The model under review builds one solid part; all positions refer to its coordinate system, in mm. A direction names the side the tool comes from. Round coordinates to 2 decimals unless told otherwise and drop trailing zeros. Order: outer loops, then holes, each group sorted by start corner. A loop starts at its lowest first (then second) coordinate and runs counter-clockwise, first axis right, second up. Notation, with made-up numbers: M -3,60.25 L 25,60.25 A31 ccw 25,93.25 Z; hole C 8.25,63 d10. An arc over 180 degrees is marked long. Use a Markdown table: item, result. Add a question column.
1. Consider section A-A on z = 5.08. Count the separate pieces of the cut face and the enclosed holes in it, then the cut area to 3 significant figures.
2. Consider section D-D on y = -3.25. State the section outline as (x, z) points, then the cut area to 3 significant figures.
3. For faces 1 (the flat face through (-5.5, 6.1, 0)), 2 (the flat face through (-18, 5.913, 10)), 3 (the flat face through (-18, 5.913, 1)), list the 3-axis set-ups (+Z, -Z, +X, -X, +Y, -Y) from which the entire face can be reached by the end or side of a thin tool; tool diameter is ignored.
4. Insertion check: P1, Ø6, axis at y = -3, z = 7, coming from the -X side; P2, Ø5, axis at x = -12, y = 2, coming from the +Z side; P3, Ø3, axis at y = 4, z = 5, coming from the -X side; P4, Ø1, axis at y = 1, z = 3, coming from the -X side. Each pin has a flat end and moves straight along its axis. Give the tip position at first contact, or say it passes through.
5. To check wall thickness, follow probe 1 along Y at (x, z) = (-2, 8); probe 2 along Y at (x, z) = (4, 1); probe 3 along X at (y, z) = (0, 0.5). State the ranges of each line that lie inside material, in increasing order.
6. Consider section B-B on y = 3. State the section outline as (x, z) points, then the cut area to 3 significant figures.
7. Consider section C-C on x = -1.5. State the section outline as (y, z) points, then the cut area to 3 significant figures.
8. The part is to be moulded in two halves that separate along X. For faces 4 (the cylindrical face through (5.74, 0.44, 5.01)), 5 (the flat face through (-18, -5.298, 1)), 6 (the cylindrical face through (5.38, 0.43, 5.01)), say which applies: +X half, -X half, draft (parallel to the pull), parting line (faces both ways), or undercut.
Autodesk Inventor part; units mm, degrees
ref_plane "YZ Plane" through (0, 0, 0) normal (1, 0, 0) x (0, 1, 0)
ref_plane "XZ Plane" through (0, 0, 0) normal (0, 1, 0) x (-1, 0, 0)
ref_plane "XY Plane" through (0, 0, 0) normal (0, 0, 1) x (1, 0, 0)
sketch "Sketch1" plane through (0, 0, 0) normal (0, 0, 1) x (1, 0, 0)
  arc A0 (0, -5.6567) -> (0, 6.271) centre (-0.2268, 0.3072) ccw
  line L0 (0, 6.271) -> (-18.4804, 6.271)
  line L1 (0, -5.6567) -> (-18.4804, -5.6567)
  line L2 (-18.122, 5.9127) -> (-0.0069, 5.9127)
  arc A1 (-0.0069, -5.2984) -> (-0.0069, 5.9127) centre (-0.2268, 0.3072) ccw
  line L3 (-0.0069, -5.2984) -> (-18.122, -5.2984)
  line L4 (-18.122, 5.9127) -> (-18.4804, 5.9127)
  line L5 (-18.4804, 6.271) -> (-18.4804, 5.9127)
  line L6 (-18.122, -5.2984) -> (-18.4804, -5.2984)
  line L7 (-18.4804, -5.6567) -> (-18.4804, -5.2984)
  point P0 (0, 0)
extrude "Extrusion1" add sketch "Sketch1" along normal blind 10.16
sketch "Sketch2" plane through (-18.4804, -5.2984, 0) normal (0, 1, 0) x (1, 0, 0)
  circle A0 centre (4.4536, -5.08) radius 0.4915
  point P0 (18.4804, 0)
extrude "Extrusion2" add sketch "Sketch2" along normal blind 11.43
fillet "Fillet1" radius 4.7625 1 edges at (-14.5182, -5.2984, 5.08)
fillet "Fillet2" radius 4.7625 1 edges at (-14.5182, 5.9127, 5.08)
sketch "Sketch3" plane through (-18.4804, -5.6567, 0) normal (0, -1, 0) x (1, 0, 0)
  circle A0 centre (4.4536, 5.08) radius 0.399
extrude "Extrusion3" cut sketch "Sketch3" against normal blind 25.4
fillet "Fillet3" radius 4.7625 1 edges at (-14.4258, 6.271, 5.08)
fillet "Fillet4" radius 4.7625 1 edges at (-14.4258, -5.6567, 5.08)
properties part number "space time"
Answer block:
| question | item | result |
|---|---|---|
| 1 | separate pieces | 2 |
| 1 | enclosed holes | 1 |
| 1 | area | 21.1 mm^2 |
| 2 | outline | C -14.03,5.08 d2.68; M 4.11,0 L 4.57,0 L 4.57,10.16 L 4.11,10.16 Z; hole C -14.03,5.08 d2.04 |
| 2 | area | 6.98 mm^2 |
| 3 | face 1 | -Z, +X, -X, +Y, -Y |
| 3 | face 2 | +Z, -X |
| 3 | face 3 | -Z, -X |
| 4 | P1 | x = -18.48 |
| 4 | P2 | z = 6.44 |
| 4 | P3 | x = -17.34 |
| 4 | P4 | x = 5.25 |
| 5 | probe 1 | -5.66 to -5.3, 5.91 to 6.27 |
| 5 | probe 2 | -3.91 to -3.38, 4 to 4.52 |
| 5 | probe 3 | 5.37 to 5.73 |
| 6 | outline | C -14.03,5.08 d1.73; M 4.69,0 L 5.1,0 L 5.1,10.16 L 4.69,10.16 Z; hole C -14.03,5.08 d1.28 |
| 6 | area | 5.18 mm^2 |
| 7 | outline | M -5.66,0 L -5.3,0 L -5.3,10.16 L -5.66,10.16 Z; M 5.91,0 L 6.27,0 L 6.27,10.16 L 5.91,10.16 Z |
| 7 | area | 7.28 mm^2 |
| 8 | face 4 | +X half |
| 8 | face 5 | draft |
| 8 | face 6 | undercut |
